from build123d import *

# Parameters (mm, degrees)
SKETCH1_W           = 130
SKETCH1_H           = 130
BOSS_EXTRUDE1_DEPTH = 5
SKETCH2_R           = 4.05
CUT_EXTRUDE1_DEPTH  = 10
FILLET1_START       = -1
FILLET1_OUTLINE_R   = 2.55
FILLET1_OUTLINE_R_2 = 2.05
FILLET1_DEPTH       = 7


with BuildPart() as part:
    # Sketch1 → Boss-Extrude1 (new body)
    with BuildSketch(Plane(origin=(0, 0, 0), x_dir=(1, 0, 0), z_dir=(0, 1, 0))):
        with Locations((65, -65)):
            Rectangle(SKETCH1_W, SKETCH1_H)
    extrude(amount=BOSS_EXTRUDE1_DEPTH)

    # Sketch2 → Cut-Extrude1 (cut)
    with BuildSketch(Plane(origin=(0, 5, 0), x_dir=(1, 0, 0), z_dir=(0, 1, 0))):
        with Locations(Location((14, -54, 0), (0, 0, 270))):
            Circle(SKETCH2_R)
        with Locations(Location((116, -54, 0), (0, 0, 270))):
            Circle(SKETCH2_R)
        with Locations(Location((116, -122, 0), (0, 0, 270))):
            Circle(SKETCH2_R)
        with Locations(Location((14, -122, 0), (0, 0, 270))):
            Circle(SKETCH2_R)
    extrude(amount=-CUT_EXTRUDE1_DEPTH, mode=Mode.SUBTRACT)

    # Fillet1: read off the stored shape, not the designer's step
    # Fillet1 outline → Fillet1 (cut)
    with BuildSketch(Plane(origin=(0, 0, 0), x_dir=(1, 0, 0), z_dir=(0, 1, 0)).offset(FILLET1_START)):
        with Locations((41.997459274, -8.5)):
            Circle(FILLET1_OUTLINE_R)
        with Locations((41.997459274, -77.5)):
            Circle(FILLET1_OUTLINE_R)
        with Locations((41.997459274, -103.5)):
            Circle(FILLET1_OUTLINE_R)
        with Locations((7.997459274, -103.5)):
            Circle(FILLET1_OUTLINE_R)
        with Locations((88.002540726, -77.5)):
            Circle(FILLET1_OUTLINE_R)
        with Locations((88.002540726, -103.5)):
            Circle(FILLET1_OUTLINE_R)
        with Locations((41.997459274, -34.5)):
            Circle(FILLET1_OUTLINE_R)
        with Locations((7.997459274, -8.5)):
            Circle(FILLET1_OUTLINE_R)
        with Locations((7.997459274, -34.5)):
            Circle(FILLET1_OUTLINE_R)
        with Locations((7.997459274, -77.5)):
            Circle(FILLET1_OUTLINE_R)
        with Locations((88.002540726, -8.5)):
            Circle(FILLET1_OUTLINE_R)
        with Locations((55, -59.941575486)):
            Circle(FILLET1_OUTLINE_R_2)
        with Locations((75, -59.941575486)):
            Circle(FILLET1_OUTLINE_R_2)
        with Locations((75, -79.941575486)):
            Circle(FILLET1_OUTLINE_R_2)
        with Locations((55, -79.941575486)):
            Circle(FILLET1_OUTLINE_R_2)
        with Locations((88.002540726, -34.5)):
            Circle(FILLET1_OUTLINE_R)
        with Locations((122.002540726, -34.5)):
            Circle(FILLET1_OUTLINE_R)
        with Locations((122.002540726, -8.5)):
            Circle(FILLET1_OUTLINE_R)
        with Locations((122.002540726, -77.5)):
            Circle(FILLET1_OUTLINE_R)
        with Locations((122.002540726, -103.5)):
            Circle(FILLET1_OUTLINE_R)
        with BuildLine():
            Line((130, -130), (130, -127))
            ThreePointArc((130, -127), (129.121320344, -129.121320344), (127, -130))
            Line((127, -130), (130, -130))
        make_face()
        with BuildLine():
            ThreePointArc((127, 0), (129.121320344, -0.878679656), (130, -3))
            Line((130, -3), (130, 0))
            Line((130, 0), (127, 0))
        make_face()
        with BuildLine():
            Line((0, -130), (3, -130))
            ThreePointArc((3, -130), (0.878679656, -129.121320344), (0, -127))
            Line((0, -127), (0, -130))
        make_face()
        with BuildLine():
            ThreePointArc((0, -3), (0.878679656, -0.878679656), (3, 0))
            Line((3, 0), (0, 0))
            Line((0, 0), (0, -3))
        make_face()
    extrude(amount=FILLET1_DEPTH, mode=Mode.SUBTRACT)


solid = part.part
Can you work these out from the model? Positions are in its coordinate system, mm. Give positions to 0.01 mm unless a question says otherwise; leave off trailing zeros. Loops run counter-clockwise (first coordinate to the right, second up) from the corner with the lowest first, then second, coordinate; pieces in that order, holes last. Notation, with made-up numbers: (60, -29) - (93, -29) arc R25 cw to (93, -6) - close; hole circle Ø8 at (38, 21). An arc over 180 degrees is marked (long way). Return JSON: item names as keys, results as strings.
1. I'm going to push a flat-ended pin straight in: pin 1 Ø12 at (x, z) = (49, 92) entering from -Y. Where does the tip first touch, or does it pass through?
Output values:
{"pin 1": "stops at y = 0"}
2. We'd pull the mould along Z, two halves only. Please class faces 1 (the face through (64, 2, 0)), 2 (the face through (7.44, 2.46, 10.99)), 3 (the face through (129.14, 2.46, 129.1)), 4 (the face through (130, 2, 66)): +Z half, -Z half, draft (parallel to the pull), parting line (faces both ways), or undercut.
Output values:
{"face 1": "-Z half", "face 2": "undercut", "face 3": "+Z half", "face 4": "draft"}
3. If I drill on line 1 (X direction, y = 2.3, z = 121.5); line 2 (Z direction, x = 12.5, y = 4.5); line 3 (Z direction, x = 118, y = 0.4), over which ranges is the centre line in solid material (lowest first)?
Output values:
{"line 1": "x = 0 to 9.98, 18.02 to 111.98, 120.02 to 130", "line 2": "z = 0 to 50.24, 57.76 to 118.24, 125.76 to 130", "line 3": "z = 0 to 50.48, 57.52 to 118.48, 125.52 to 130"}
4. I want a section at B-B on z = 103.5. Please give me the cut outline in (x, y), and give its area (3 significant figures).
Output values:
{"outline": "(0, 0) - (5.45, 0) - (5.45, 5) - (0, 5) - close; (10.55, 0) - (39.45, 0) - (39.45, 5) - (10.55, 5) - close; (44.55, 0) - (85.45, 0) - (85.45, 5) - (44.55, 5) - close; (90.55, 0) - (119.45, 0) - (119.45, 5) - (90.55, 5) - close; (124.55, 0) - (130, 0) - (130, 5) - (124.55, 5) - close", "area": "548 mm²"}
5. I want a section at A-A on x = 75. Please give me the cut outline in (y, z).
Output values:
{"outline": "(0, 0) - (5, 0) - (5, 57.89) - (0, 57.89) - close; (0, 61.99) - (5, 61.99) - (5, 77.89) - (0, 77.89) - close; (0, 81.99) - (5, 81.99) - (5, 130) - (0, 130) - close"}
6. I want a section at D-D on z = 54. Please give me the cut outline in (x, y).
Output values:
{"outline": "(0, 0) - (9.95, 0) - (9.95, 5) - (0, 5) - close; (18.05, 0) - (111.95, 0) - (111.95, 5) - (18.05, 5) - close; (120.05, 0) - (130, 0) - (130, 5) - (120.05, 5) - close"}
7. I want a section at C-C on x = 88. Please give me the cut outline in (y, z), and give its area (3 significant figures).
Output values:
{"outline": "(0, 0) - (5, 0) - (5, 5.95) - (0, 5.95) - close; (0, 11.05) - (5, 11.05) - (5, 31.95) - (0, 31.95) - close; (0, 37.05) - (5, 37.05) - (5, 74.95) - (0, 74.95) - close; (0, 80.05) - (5, 80.05) - (5, 100.95) - (0, 100.95) - close; (0, 106.05) - (5, 106.05) - (5, 130) - (0, 130) - close", "area": "548 mm²"}
